The model under review builds one solid part; all positions refer to its coordinate system, in mm. Face numbers are marked on the shaded views. A direction names the side the tool comes from. Coordinates: 2 decimals unless noted, no trailing zeros. Loops run counter-clockwise (first coordinate to the right, second up) from the corner with the lowest first, then second, coordinate; pieces in that order, holes last. Notation, with made-up numbers: M 44.25,16 L 81.25,16 A27 ccw 81.25,51 Z; hole C 51,-32.5 d7. An arc over 180 degrees is marked long. Use CSV: the item, a comma, the result in double quotes. Start each with the question number.
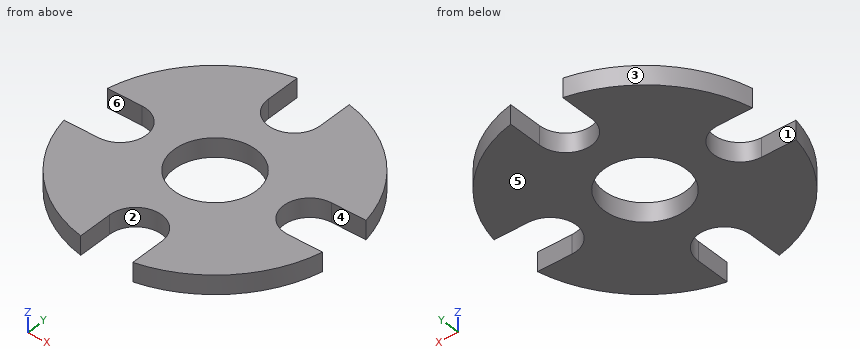
from build123d import *

# Parameters (mm, degrees)
BOSS_EXTRUDE1_DEPTH = 50.8
SKETCH2_R           = 110
CUT_EXTRUDE1_DEPTH  = 495.80363782


with BuildPart() as part:
    # Sketch1 → Boss-Extrude1 (new body)
    with BuildSketch(Plane.XY):
        with BuildLine():
            ThreePointArc((348.030171106, 70), (251.022907321, 251.022907321), (70, 348.030171106))
            Line((70, 348.030171106), (70, 255))
            ThreePointArc((70, 255), (0, 185), (-70, 255))
            Line((-70, 255), (-70, 348.030171106))
            ThreePointArc((-70, 348.030171106), (-251.022907321, 251.022907321), (-348.030171106, 70))
            Line((-348.030171106, 70), (-255, 70))
            ThreePointArc((-255, 70), (-185, 0), (-255, -70))
            Line((-255, -70), (-348.030171106, -70))
            ThreePointArc((-348.030171106, -70), (-251.022907321, -251.022907321), (-70, -348.030171106))
            Line((-70, -348.030171106), (-70, -255))
            ThreePointArc((-70, -255), (0, -185), (70, -255))
            Line((70, -255), (70, -348.030171106))
            ThreePointArc((70, -348.030171106), (251.022907321, -251.022907321), (348.030171106, -70))
            Line((348.030171106, -70), (255, -70))
            ThreePointArc((255, -70), (185, 0), (255, 70))
            Line((255, 70), (348.030171106, 70))
        make_face()
    extrude(amount=BOSS_EXTRUDE1_DEPTH)

    # Sketch2 → Cut-Extrude1 (cut, through all)
    with BuildSketch(Plane.XY.offset(50.8)):
        Circle(SKETCH2_R)
    extrude(amount=-CUT_EXTRUDE1_DEPTH, mode=Mode.SUBTRACT)


solid = part.part
1. To check wall thickness, follow line 1 along Y through (x, z) = (0, 26); line 2 along Y through (x, z) = (19.5, 8.5); line 3 along X through (y, z) = (-27.5, 36.5). State the ranges of each line that lie inside material, in increasing order.
2. Add section D-D (y = 122.5). Write out the cut boundary in (x, z), plus the area to 3 significant figures.
3. Add section B-B (x = -49.5). Write out the cut boundary in (y, z), plus the area to 3 significant figures.
4. Add section C-C (y = 24). Write out the cut boundary in (x, z), plus the area to 3 significant figures.
5. Add section A-A (z = 19). Write out the cut boundary in (x, y), plus the area to 3 significant figures.
6. For the marked faces 4, 5 and 6, list the 3-axis set-ups (+Z, -Z, +X, -X, +Y, -Y) from which the entire face can be reached by the end or side of a thin tool; tool diameter is ignored.
7. Draft analysis for pull direction X (two halves, no side actions). For the marked faces 1, 2 and 3, state which applies: released by +X, released by -X, zero draft, split by the parting line, or undercut.
8. Insertion check: pin 1 Ø15 at (y, z) = (304, 25.5) entering from -X; pin 2 Ø8 at (x, z) = (10, 45.5) entering from +Y; pin 3 Ø10 at (x, z) = (46, 28.5) entering from -Y; pin 4 Ø12 at (x, y) = (208, -60.5) entering from -Z. Each pin has a flat end and moves straight along its axis. Give the tip position at first contact, or say it passes through.
Solved:
1,line 1,"y = -185 to -110, 110 to 185"
1,line 2,"y = -187.77 to -108.26, 108.26 to 187.77"
1,line 3,"x = -190.63 to -106.51, 106.51 to 190.63"
2,outline,"M -333.19,0 L 333.19,0 L 333.19,50.8 L -333.19,50.8 Z"
2,area,"33,900 mm^2"
3,outline,"M -205.51,0 L -98.23,0 L -98.23,50.8 L -205.51,50.8 Z; M 98.23,0 L 205.51,0 L 205.51,50.8 L 98.23,50.8 Z"
3,area,"10,900 mm^2"
4,outline,"M -189.24,0 L -107.35,0 L -107.35,50.8 L -189.24,50.8 Z; M 107.35,0 L 189.24,0 L 189.24,50.8 L 107.35,50.8 Z"
4,area,"8,320 mm^2"
5,outline,"M -348.03,-70 A355 ccw -70,-348.03 L -70,-255 A70 cw 70,-255 L 70,-348.03 A355 ccw 348.03,-70 L 255,-70 A70 cw 255,70 L 348.03,70 A355 ccw 70,348.03 L 70,255 A70 cw -70,255 L -70,348.03 A355 ccw -348.03,70 L -255,70 A70 cw -255,-70 Z; hole C 0,0 d220"
5,area,"272,000 mm^2"
6,face 4,"+Z, -Z, +X"
6,face 5,"-Z, +X, -X, +Y, -Y"
6,face 6,"+Z, -Z, -X"
7,face 1,"zero draft"
7,face 2,"undercut"
7,face 3,"released by -X"
8,pin 1,"stops at x = -195.22"
8,pin 2,"stops at y = 186.41"
8,pin 3,"stops at y = -207.05"
8,pin 4,"stops at z = 0"
